Check sheet for the modelled part. Datum: model origin and axes. Units: mm. A direction names the side the tool comes from. Give positions to 0.01 mm unless a question says otherwise; leave off trailing zeros. Loops run counter-clockwise (first coordinate to the right, second up) from the corner with the lowest first, then second, coordinate; pieces in that order, holes last. Notation, with made-up numbers: (80, -16.5) - (138, -16.5) arc R26 ccw to (138, 19.5) - close; hole circle Ø10 at (-29, 50). An arc over 180 degrees is marked (long way). Use CSV: the item, a comma, the result in double quotes.
Autodesk Inventor part; units mm, degrees
ref_plane "YZ Plane" through (0, 0, 0) normal (1, 0, 0) x (0, 1, 0)
ref_plane "XZ Plane" through (0, 0, 0) normal (0, 1, 0) x (-1, 0, 0)
ref_plane "XY Plane" through (0, 0, 0) normal (0, 0, 1) x (1, 0, 0)
sketch "Sketch1" plane through (0, 0, 0) normal (0, 0, 1) x (1, 0, 0)
  line L0 (3.5929, 6.223) -> (7.1857, 0)
  line L1 (7.1857, 0) -> (3.5929, -6.223)
  line L2 (3.5929, -6.223) -> (-3.5929, -6.223)
  line L3 (-3.5929, -6.223) -> (-7.1857, 0)
  line L4 (-7.1857, 0) -> (-3.5929, 6.223)
  line L5 (-3.5929, 6.223) -> (3.5929, 6.223)
  line L6 (2.823, 4.8895) -> (5.6459, 0)
  line L7 (5.6459, 0) -> (2.823, -4.8895)
  line L8 (2.823, -4.8895) -> (-2.823, -4.8895)
  line L9 (-2.823, -4.8895) -> (-5.6459, 0)
  line L10 (-5.6459, 0) -> (-2.823, 4.8895)
  line L11 (-2.823, 4.8895) -> (2.823, 4.8895)
  point P0 (0, 0)
  point P1 (0, 0)
  point P2 (0, 0)
  dimension "d0" = 12.446
  dimension "d1" = 9.779
extrude "Extrusion1" add sketch "Sketch1" along normal mid plane 15.875
properties part number "1-2 TO 3-8 ADAPTER" material "ABS Plastic"
1. Sectioned sample at A-A, the plane x = -2.5. Record the boundary of the cut face in (y, z), and give its area (3 significant figures).
Completed:
outline,"(-6.22, -7.94) - (-4.89, -7.94) - (-4.89, 7.94) - (-6.22, 7.94) - close; (4.89, -7.94) - (6.22, -7.94) - (6.22, 7.94) - (4.89, 7.94) - close"
area,"42.3 mm²"
2. Sectioned sample at B-B, the plane y = 1.5. Record the boundary of the cut face in (x, z).
Completed:
outline,"(-6.32, -7.94) - (-4.78, -7.94) - (-4.78, 7.94) - (-6.32, 7.94) - close; (4.78, -7.94) - (6.32, -7.94) - (6.32, 7.94) - (4.78, 7.94) - close"
3. Set-up check for faces 4 (the face through (4.254, -2.411, -0.111)), 5 (the face through (0, 6.223, 0)): record each of +Z, -Z, +X, -X, +Y, -Y from which the full face is reachable in a straight line by a thin tool's end or side.
Completed:
face 4,"+Z, -Z"
face 5,"+Z, -Z, +X, -X, +Y"
4. Sectioned sample at C-C, the plane z = -4.75. Record the boundary of the cut face in (x, y), and give its area (3 significant figures).
Completed:
outline,"(-7.19, 0) - (-3.59, -6.22) - (3.59, -6.22) - (7.19, 0) - (3.59, 6.22) - (-3.59, 6.22) - close; hole (-5.65, 0) - (-2.82, -4.89) - (2.82, -4.89) - (5.65, 0) - (2.82, 4.89) - (-2.82, 4.89) - close"
area,"51.3 mm²"
5. Go/stop test with a flat-tipped pin: pin 1 Ø1.5 at (x, z) = (4.5, 1.5) entering from +Y. Record where the tip stops, or that it passes through.
Completed:
pin 1,"stops at y = 5.95"
6. Release check for a two-part mould opening along Y. For faces 1 (the face through (4, -4, 7.938)), 2 (the face through (0, 4.89, 0)), 3 (the face through (-5.414, 3.068, -0.111)) record: released by +Y, released by -Y, zero draft, split by the parting line, or undercut.
Completed:
face 1,"zero draft"
face 2,"undercut"
face 3,"released by +Y"
7. Scan lines: line 1 along Y through (x, z) = (0, 3.75); line 2 along X through (y, z) = (0.25, -6.75); line 3 along Y through (x, z) = (-3, 0.5). Record each from-to range of solid material in increasing order.
Completed:
line 1,"y = -6.22 to -4.89, 4.89 to 6.22"
line 2,"x = -7.04 to -5.5, 5.5 to 7.04"
line 3,"y = -6.22 to -4.58, 4.58 to 6.22"
